Verification items for this drawing (mm, ordinates from the low corner). Round coordinates to 2 decimals unless told otherwise and drop trailing zeros. Write each loop counter-clockwise with the first axis right and the second up, starting at its lowest first coordinate (ties: lowest second). Pieces come first, ordered by that corner, then holes. Notation, with made-up numbers: (-10.5, -26) -> (47.5, -26) arc R20 cw to (47.5, -19) -> close; hole circle Ø2 at (88.25, -24.75). An arc over 180 degrees is marked (long way). One line per question, with ' | ' between items.
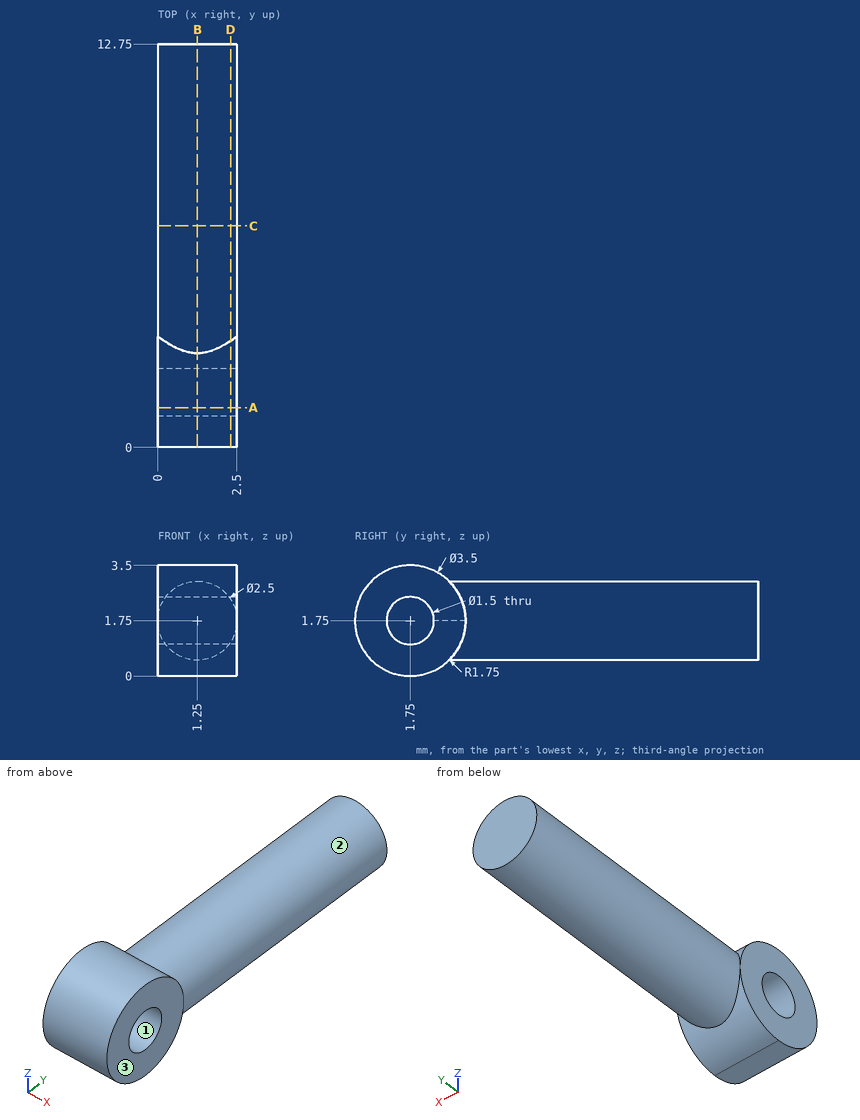
(1) Sectioned sample at B-B on x = 1.25. Record the cut outline in (y, z).
Resolved:
outline: (2.97, 0.5) -> (12.75, 0.5) -> (12.75, 3) -> (2.97, 3) arc R1.75 ccw (long way) to start; hole circle Ø1.5 at (1.75, 1.75)
(2) Sectioned sample at A-A on y = 1.25. Record the cut outline in (x, z).
Resolved:
outline: (0, 0.07) -> (2.5, 0.07) -> (2.5, 1.19) -> (0, 1.19) -> close; (0, 2.31) -> (2.5, 2.31) -> (2.5, 3.43) -> (0, 3.43) -> close
(3) Sectioned sample at D-D on x = 2.3. Record the cut outline in (y, z).
Resolved:
outline: (3.36, 1.07) -> (12.75, 1.07) -> (12.75, 2.43) -> (3.36, 2.43) arc R1.75 ccw (long way) to start; hole circle Ø1.5 at (1.75, 1.75)
(4) Go/stop test with a flat-tipped pin: pin 1 (1 mm diameter, centred on x = 1, y = 6.5, fed in from +Z). Record where the tip stops, or that it passes through.
Resolved:
pin 1: stops at z = 3
(5) Material ranges on line 1 (Y direction, x = 1.5, z = 1.6); line 2 (Z direction, x = 0.85, y = 7); line 3 (X direction, y = 9, z = 1.5), recorded low to high.
Resolved:
line 1: y = 0.01 to 1.02, 2.48 to 12.75 | line 2: z = 0.57 to 2.93 | line 3: x = 0.03 to 2.47
(6) Draft check along Z on the marked faces 1, 2 and 3. Enter one of: +Z half, -Z half, draft (parallel to the pull), parting line (faces both ways), or undercut.
Resolved:
face 1: undercut | face 2: parting line | face 3: draft
(7) Sectioned sample at C-C on y = 7. Record the cut outline in (x, z), then the cut area to 3 significant figures.
Resolved:
outline: circle Ø2.5 at (1.25, 1.75) | area: 4.91 mm2
